Solid Edge part; units mm, degrees
sketch "Sketch1" plane through (0, 0, 0) normal (0, 0, 1) x (1, 0, 0)
  line L0 (-1, 21.921) -> (23.4451, 4.8043)
  line L1 (22.298, 3.166) -> (23.4451, 4.8043)
  line L2 (1, 18.079) -> (22.298, 3.166)
  line L3 (1, -2.921) -> (1, 18.079)
  line L4 (-1, -2.921) -> (1, -2.921)
  line L5 (-1, -2.921) -> (-1, 21.921)
  line L6 (-2, 23.842) -> (24.8378, 5.0499)
  line L7 (22.5435, 1.7733) -> (24.8378, 5.0499)
  line L8 (2, 16.158) -> (22.5435, 1.7733)
  line L9 (2, -3.921) -> (2, 16.158)
  line L10 (2, -3.921) -> (-2, -3.921)
  line L11 (-2, -3.921) -> (-2, 23.842)
extrude "Protrusion1" add sketch "Sketch1" along normal blind 20
sketch "Sketch2" plane through (11.649, 10.6225, 10) normal (0.5735764, 0.819152, 0) x (0.819152, -0.5735764, 0)
  line L0 (-18.7629, -30) -> (14, -10)
  line L1 (14, -10) -> (-18.7629, -10)
  line L2 (-18.7629, -10) -> (-18.7629, -30)
extrude "ProtrusioneEstrusa_4" add sketch "Sketch2" against normal up to vertex (1 mm away) and the other way blind 0.3
sketch "Sketch3" plane through (11.4189, 13.3401, 20) normal (0, 0, 1) x (-0.819152, 0.5735764, 0)
  line L0 (-15.7472, -0.9059) -> (-15.7472, 3.0941)
  line L1 (-15.7472, 3.0941) -> (9.3318, 3.0941)
  line L2 (9.3318, 3.0941) -> (-2.185, 19.5419)
  line L3 (-2.185, 19.5419) -> (1.0916, 21.8362)
  line L4 (1.0916, 21.8362) -> (17.0158, -0.9059)
  line L5 (17.0158, -0.9059) -> (-15.7472, -0.9059)
extrude "ProtrusioneEstrusa_5" add sketch "Sketch3" against normal blind 1.2
sketch "Sketch4" plane through (-3.1472, 20.2946, 20) normal (0, 0, -1) x (-0.819152, 0.5735764, 0)
  line L0 (-0.7955, 0.8638) -> (1.095, 0.8638)
  line L1 (1.095, 0.8638) -> (1.095, -0.4362)
  line L2 (1.095, -0.4362) -> (-1.7058, -0.4362)
  line L3 (-1.7058, -0.4362) -> (-0.7955, 0.8638)
extrude "ScavoEstrusione_3" cut sketch "Sketch4" against normal blind 20.5093 and the other way blind 1.027
Work out the finished part from the listing and answer in its coordinate system (mm). A direction names the side the tool comes from. Give positions to 0.01 mm unless a question says otherwise; leave off trailing zeros. Loops run counter-clockwise (first coordinate to the right, second up) from the corner with the lowest first, then second, coordinate; pieces in that order, holes last. Notation, with made-up numbers: (-28.5, -6.5) -> (-5.5, -6.5) arc R19 ccw to (-5.5, 0.5) -> close; hole circle Ø6 at (6.5, -25). An arc over 180 degrees is marked (long way). Use a Markdown table: item, result. Add a question column.
1) The part is cut by section A-A, the plane y = 4. Determine the outline of the cut face in (x, z).
2) The part is cut by section C-C, the plane z = 15. Determine the outline of the cut face in (x, y), plus the area to 3 significant figures.
3) The part is cut by section D-D, the plane y = 17. Determine the outline of the cut face in (x, z).
4) Consider line 1 along X through (y, z) = (5, 10.5); line 2 along X through (y, z) = (12.5, 5); line 3 along X through (y, z) = (-3, 7). Determine where each line is inside the solid, lowest interval first.
5) Each of these flat-tipped pins is pushed along its axis until it touches: P1, Ø8, axis at x = 10.5, z = 6.5, coming from the +Y side; P2, Ø2, axis at x = 1, y = 2, coming from the +Z side; P3, Ø12, axis at x = 21.5, z = 10, coming from the -Y side; P4, Ø5, axis at y = 7, z = 16, coming from the +X side. Where does it stop, or does it pass through?
6) The part is cut by section B-B, the plane x = 18.25. Determine the outline of the cut face in (y, z).
7) Which of the six approach directions +Z, -Z, +X, -X, +Y, -Y give full straight-line access (tool end or side, diameter ignored) to faces 1 (the flat face through (1, 7, 9)), 2 (the flat face through (2, 6, 10)), 3 (the flat face through (11, 13, 20))?
8) For a pull along X with two mould halves and no side action, classify faces 4 (the flat face through (0, 8, 20)), 5 (the flat face through (10.1, 11.291, 29.555)), 6 (the flat face through (11.5, 10.727, 9.268)) as +X half, -X half, draft (parallel to the pull), parting line (faces both ways), or undercut.
Reported:
| question | item | result |
|---|---|---|
| 1 | outline | (-2, 0) -> (-1, 0) -> (-1, 18.8) -> (1, 18.8) -> (1, 0) -> (2, 0) -> (2, 20) -> (-2, 20) -> close; (19.36, 0) -> (21.11, 0) -> (21.11, 18.8) -> (22.88, 18.8) -> (22.88, 0) -> (24.1, 0) -> (24.1, 20) -> (21.63, 20) -> (21.63, 21.24) -> (19.36, 22.37) -> close |
| 2 | outline | (-2, -3.92) -> (2, -3.92) -> (2, 16.16) -> (22.54, 1.77) -> (24.84, 5.05) -> (-2, 23.84) -> close; hole (-1, -2.92) -> (1, -2.92) -> (1, 18.08) -> (22.3, 3.17) -> (23.45, 4.8) -> (-1, 21.92) -> close |
| 2 | area | 110 mm^2 |
| 3 | outline | (-2, 0) -> (-1, 0) -> (-1, 18.8) -> (1, 18.8) -> (1, 0) -> (2.54, 0) -> (2.54, 18.8) -> (6.03, 18.8) -> (6.03, 0) -> (7.77, 0) -> (7.77, 20) -> (3.06, 20) -> (3.06, 35.07) -> (0.8, 36.21) -> (0.8, 20) -> (-2, 20) -> close |
| 4 | line 1 | x = -2 to -1, 1 to 2, 17.94 to 19.68, 23.17 to 24.8 |
| 4 | line 2 | x = -2 to -1, 1 to 2, 7.22 to 8.97, 12.45 to 14.2 |
| 4 | line 3 | x = -2 to 2 |
| 5 | P1 | stops at y = 17.89 |
| 5 | P2 | stops at z = 20 |
| 5 | P3 | stops at y = 1.77 |
| 5 | P4 | stops at x = 24.84 |
| 6 | outline | (4.78, 0) -> (6, 0) -> (6, 18.8) -> (8.44, 18.8) -> (8.44, 0) -> (9.66, 0) -> (9.66, 20) -> (6.37, 20) -> (6.37, 23.76) -> (4.78, 23.2) -> close |
| 7 | face 1 | -Z |
| 7 | face 2 | +Z, -Z, -Y |
| 7 | face 3 | +Z, +X, +Y |
| 8 | face 4 | draft |
| 8 | face 5 | +X half |
| 8 | face 6 | undercut |
